Input: part model. Units: mm. Frame: model coordinates. A direction names the side the tool comes from. Coordinates: 2 decimals unless noted, no trailing zeros. Order: outer loops, then holes, each group sorted by start corner. A loop starts at its lowest first (then second) coordinate and runs counter-clockwise, first axis right, second up. Notation, with made-up numbers: (84, 1.25) -> (137, 1.25) arc R23 cw to (137, 31.25) -> close; hole circle Ø7 at (22, 52.25). An arc over 180 degrees is marked (long way). Use CSV: the item, a comma, the result in double quotes. Start each with the question number.
```python
from build123d import *

# Parameters (mm, degrees)
SKETCH_1_W                   = 66
SKETCH_1_H                   = 68
EXTRUDE_1_DEPTH              = 3
CUT_EXTRUDE_START            = 3
SKETCH_1_3_W                 = 54
SKETCH_1_3_H                 = 54
CUT_EXTRUDE_1_DEPTH          = 1
HOLE_WIZARD_M3_1_D           = 3.2
HOLE_WIZARD_M3_1_CSINK_D     = 6.3
HOLE_WIZARD_M3_1_CSINK_ANGLE = 90
M3X0_5_1_D                   = 2.5
M3X0_5_1_DEPTH               = 8.5
M3X0_5_1_CBORE_D             = 3
M3X0_5_1_CBORE_DEPTH         = 6
M3X0_5_1_TIP                 = 0.751075774


with BuildPart() as part:
    # ｽｹｯﾁ1 → ﾎﾞｽ - 押し出し1 (new, symmetric)
    with BuildSketch(Plane.XY):
        Rectangle(SKETCH_1_W, SKETCH_1_H)
    extrude(amount=EXTRUDE_1_DEPTH, both=True)

    # ｽｹｯﾁ1<3> → ｶｯﾄ - 押し出し1 (cut)
    with BuildSketch(Plane.XY.offset(CUT_EXTRUDE_START)):
        Polygon((-27, 34), (-33, 34), (-33, -34), (-27, -34), (-27, -33), (27, -33), (27, -34), (33, -34), (33, 34), (27, 34), (27, 33), (-27, 33), align=None)
        Rectangle(SKETCH_1_3_W, SKETCH_1_3_H, mode=Mode.SUBTRACT)
    extrude(amount=-CUT_EXTRUDE_1_DEPTH, mode=Mode.SUBTRACT)

    # M3 丸皿ねじ用皿穴1 (through all)
    with Locations(Plane(origin=(24, 30, -3), x_dir=(-1, 0, 0), z_dir=(0, 0, -1))):
        with Locations((0, 0), (24, 0), (48, 0), (48, -60), (24, -60), (0, -60), (-6, -6), (-6, -54), (54, -54), (54, -6)):
            CounterSinkHole(HOLE_WIZARD_M3_1_D / 2, HOLE_WIZARD_M3_1_CSINK_D / 2, counter_sink_angle=HOLE_WIZARD_M3_1_CSINK_ANGLE)

    # M3x0.5 ねじ穴1
    with Locations(Plane(origin=(-15, -34, 0), x_dir=(-1, 0, 0), z_dir=(0, -1, 0))):
        with Locations((0, 0), (-30, 0)):
            CounterBoreHole(M3X0_5_1_D / 2, M3X0_5_1_CBORE_D / 2, M3X0_5_1_CBORE_DEPTH, depth=M3X0_5_1_DEPTH)
            with Locations((0, 0, -(M3X0_5_1_DEPTH + M3X0_5_1_TIP / 2))):  # 118° drill point
                Cone(0, M3X0_5_1_D / 2, M3X0_5_1_TIP, mode=Mode.SUBTRACT)


solid = part.part
```
1. Contact query for flat-ended pins moving along their axis: P1, Ø4, axis at x = -24, y = -30, coming from the -Z side; P2, Ø5, axis at x = -30, y = 24, coming from the +Z side; P3, Ø0.8, axis at y = -33.5, z = 2.5, coming from the -X side. Output: stop coordinate, or through.
2. Material intervals for line 1 along Y through (x, z) = (24, -0.4); line 2 along X through (y, z) = (-30, 0.2); line 3 along Y through (x, z) = (1, 2.7), sorted ascending.
3. Section D-D on y = 0. Return loops of the section in (x, z), then the cut area to 3 significant figures.
4. Section C-C on x = -9. Return loops of the section in (y, z), then the cut area to 3 significant figures.
5. Section B-B on x = 30. Return loops of the section in (y, z), then the cut area to 3 significant figures.
6. Access query for faces 5 (the face through (16.5, -31.04, -0.07)), 6 (the face through (-0.208, -28.414, 0.299)). Directions: +Z, -Z, +X, -X, +Y, -Y. A direction counts if a zero-diameter tool reaches every point of the face in a straight line with its end or side. Return the directions, or none.
7. Section A-A on y = -30. Return loops of the section in (x, z), then the cut area to 3 significant figures.
8. Pull-direction query (X, two-part tool) for faces 1 (the face through (14.8, -24.88, 0.08)), 2 (the face through (-29, 3, 2)), 3 (the face through (33, 0, 0)), 4 (the face through (28.82, -22.92, 0.3)); classes: released by +X, released by -X, zero draft, split by the parting line, or undercut.
Values follow:
1,P1,"stops at z = -1.85"
1,P2,"stops at z = 2"
1,P3,"stops at x = -27"
2,line 1,"y = -34 to -31.6, -28.4 to 28.4, 31.6 to 34"
2,line 2,"x = -33 to -25.6, -22.4 to -16.49, -13.51 to -1.6, 1.6 to 13.51, 16.49 to 22.4, 25.6 to 33"
2,line 3,"y = -34 to -33, -27 to 27, 33 to 34"
3,outline,"(-33, -3) -> (33, -3) -> (33, 2) -> (27, 2) -> (27, 3) -> (-27, 3) -> (-27, 2) -> (-33, 2) -> close"
3,area,"384 mm2"
4,outline,"(-34, -3) -> (34, -3) -> (34, 3) -> (33, 3) -> (33, 2) -> (27, 2) -> (27, 3) -> (-27, 3) -> (-27, 2) -> (-33, 2) -> (-33, 3) -> (-34, 3) -> close"
4,area,"396 mm2"
5,outline,"(-34, -3) -> (-27.15, -3) -> (-25.6, -1.45) -> (-25.6, 2) -> (-34, 2) -> close; (-22.4, -1.45) -> (-20.85, -3) -> (20.85, -3) -> (22.4, -1.45) -> (22.4, 2) -> (-22.4, 2) -> close; (25.6, -1.45) -> (27.15, -3) -> (34, -3) -> (34, 2) -> (25.6, 2) -> close"
5,area,"303 mm2"
6,face 5,"-Y"
6,face 6,"+Z, -Z"
7,outline,"(-33, -3) -> (-27.15, -3) -> (-25.6, -1.45) -> (-25.6, 2) -> (-33, 2) -> close; (-22.4, -1.45) -> (-20.85, -3) -> (-3.15, -3) -> (-1.6, -1.45) -> (-1.6, 2) -> (-22.4, 2) -> close; (1.6, -1.45) -> (3.15, -3) -> (20.85, -3) -> (22.4, -1.45) -> (22.4, 2) -> (1.6, 2) -> close; (25.6, -1.45) -> (27.15, -3) -> (33, -3) -> (33, 2) -> (25.6, 2) -> close; hole circle Ø3 at (-15, 0); hole circle Ø3 at (15, 0)"
7,area,"261 mm2"
8,face 1,"undercut"
8,face 2,"zero draft"
8,face 3,"released by +X"
8,face 4,"undercut"
